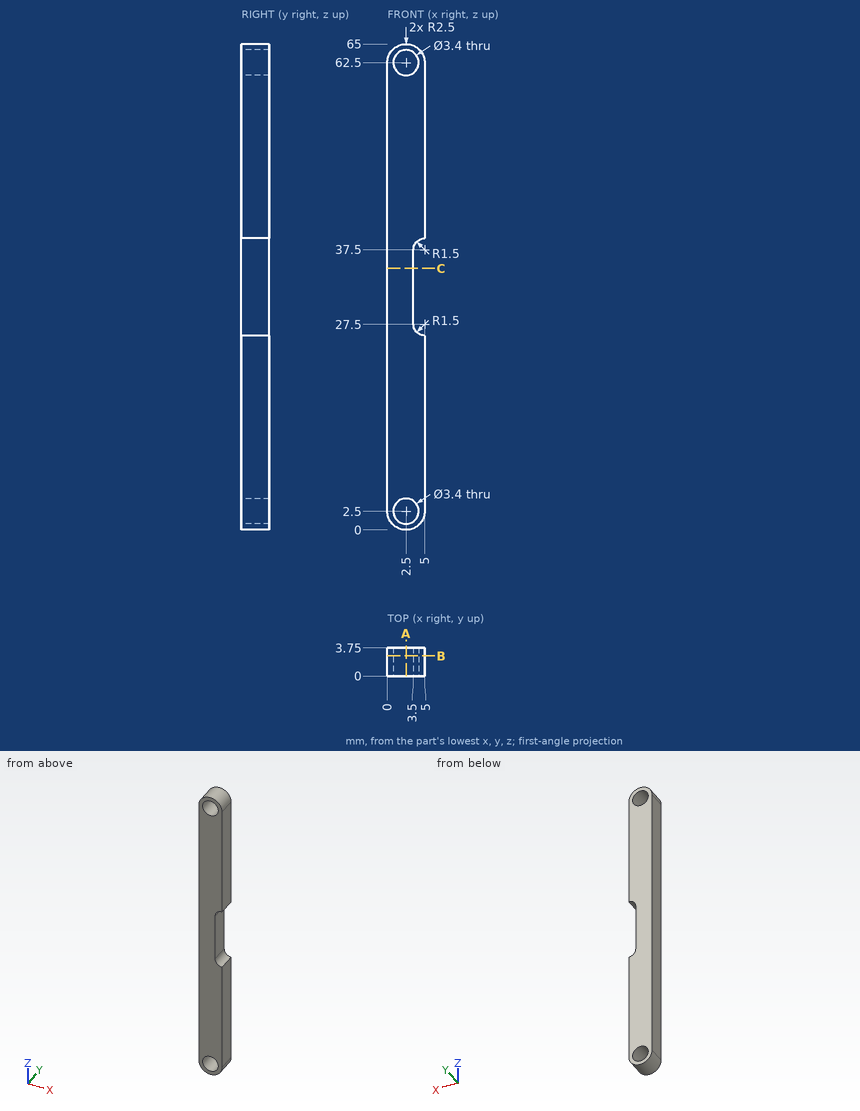
The drawing under review shows one solid part. Ordinate dimensions are in mm from its lowest x, y, z. Coordinates: 2 decimals unless noted, no trailing zeros. Write each loop counter-clockwise with the first axis right and the second up, starting at its lowest first coordinate (ties: lowest second). Pieces come first, ordered by that corner, then holes.
1) To check wall thickness, follow L1, parallel to Z at x = 2.5, y = 2.65; L2, parallel to Z at x = 2.05, y = 2.5; L3, parallel to Z at x = 4.05, y = 1. State the ranges of each line that lie inside material, in increasing order.
2) Add section C-C (z = 35). Write out the cut boundary in (x, y), plus the area to 3 significant figures.
3) Insertion check: pin 1 (1.9 mm diameter, centred on y = 1, z = 30.5, fed in from +X); pin 2 (2 mm diameter, centred on x = 2.5, z = 62.5, fed in from +Y). Each pin has a flat end and moves straight along its axis. Give the tip position at first contact, or say it passes through.
4) Add section B-B (y = 2.7). Write out the cut boundary in (x, z), plus the area to 3 significant figures.
5) Add section A-A (x = 2.5). Write out the cut boundary in (y, z).
Check result:
1. L1: z = 0 to 0.8, 4.2 to 60.8, 64.2 to 65
1. L2: z = 0.04 to 0.86, 4.14 to 60.86, 64.14 to 64.96
1. L3: z = 0.54 to 1.8, 3.2 to 26.34, 38.66 to 61.8, 63.2 to 64.46
2. outline: (0, 0) - (3.5, 0) - (3.5, 3.75) - (0, 3.75) - close
2. area: 13.1 mm2
3. pin 1: stops at x = 3.5
3. pin 2: passes through
4. outline: (0, 2.5) arc R2.5 ccw to (5, 2.5) - (5, 26) arc R1.5 cw to (3.5, 27.5) - (3.5, 37.5) arc R1.5 cw to (5, 39) - (5, 62.5) arc R2.5 ccw to (0, 62.5) - close; hole circle Ø3.4 at (2.5, 2.5); hole circle Ø3.4 at (2.5, 62.5)
4. area: 283 mm2
5. outline: (0, 0) - (3.75, 0) - (3.75, 0.8) - (0, 0.8) - close; (0, 4.2) - (3.75, 4.2) - (3.75, 60.8) - (0, 60.8) - close; (0, 64.2) - (3.75, 64.2) - (3.75, 65) - (0, 65) - close
